from build123d import *

# Parameters (mm, degrees)
F3_D     = 4.5
F3_DEPTH = 7.4
F3_TIP   = 1.3519363928


with BuildPart() as f1:
    # F0 (on Front) → F1 (revolve)
    with BuildSketch(Plane.XZ):
        Polygon((0, 7.5), (-10, 7.5), (-10, 0), (12, 0), (12, 2.5), (0, 2.5), align=None)
    revolve(axis=Axis((1, 0, 0), (1, 0, 0)))

    # F3
    with Locations(Plane(origin=(-10, 0, 0), x_dir=(0, -1, 0), z_dir=(-1, 0, 0))):
        with Locations((0, 0)):
            Hole(F3_D / 2, depth=F3_DEPTH)
            with Locations((0, 0, -(F3_DEPTH + F3_TIP / 2))):  # 118° drill point
                Cone(0, F3_D / 2, F3_TIP, mode=Mode.SUBTRACT)


solid = f1.part
Verification items for the finished model (mm, model axes). A direction names the side the tool comes from. Give positions to 0.01 mm unless a question says otherwise; leave off trailing zeros. Order: outer loops, then holes, each group sorted by start corner. A loop starts at its lowest first (then second) coordinate and runs counter-clockwise, first axis right, second up. Notation, with made-up numbers: M 0.5,65.25 L 17.5,65.25 A14 ccw 17.5,89.25 Z; hole C 7,-4 d10. An arc over 180 degrees is marked long. Use one line per item in the form item = value. Start each with the question number.
Q1. Access from +Z, -Z, +X, -X, +Y, -Y to the whole of each face (thin tool, end or side, straight path). Record for faces 1 (the cylindrical face through (5.92, 2.44, -0.54)), 2 (the cylindrical face through (-6.25, -0.29, 2.23)), 3 (the flat face through (12, 0, 0)).
Q2. Scan lines: line 1 along Z through (x, y) = (-7, 0); line 2 along X through (y, z) = (-3, 4.75). Record each from-to range of solid material in increasing order. Write a range as [from, to].
Q3. Mould release check, pull along Z, two halves, no side actions. Record for faces 4 (the cylindrical face through (-5.07, -0.33, -7.493)), 5 (the conical face through (-1.48, 0.08, -0.38)), 6 (the flat face through (0, -2, 2)): +Z half, -Z half, draft (parallel to the pull), parting line (faces both ways), or undercut.
Q4. Section check A-A (x = -3.75). Enter the section's corners in (y, z), then the cut area to 3 significant figures.
Q5. Go/stop test with flat-tipped pins: pin 1 Ø3.5 at (y, z) = (0, 0) entering from -X; pin 2 Ø1.5 at (y, z) = (5, 3.5) entering from +X; pin 3 Ø5 at (x, y) = (0, -0.5) entering from +Z; pin 4 Ø1 at (x, y) = (9, 2) entering from -Z. Record where each tip stops, or that it passes through.
Q6. Section check C-C (x = 5). Enter the section's corners in (y, z).
Q7. Section check B-B (y = -4.5). Enter the section's corners in (x, z).
Q8. Section check D-D (z = -6.25). Enter the section's corners in (x, y).
Evaluation:
q1.face_1 = +X
q1.face_2 = -X
q1.face_3 = +Z, -Z, +X, +Y, -Y
q2.line_1 = [-7.5, -2.25], [2.25, 7.5]
q2.line_2 = [-10, 0]
q3.face_4 = parting line
q3.face_5 = undercut
q3.face_6 = draft
q4.outline = C 0,0 d15; hole C 0,0 d4.5
q4.area = 161 mm2
q5.pin_1 = -2.3
q5.pin_2 = 0
q5.pin_3 = 7.5
q5.pin_4 = -2
q6.outline = C 0,0 d5
q7.outline = M -10,-6 L 0,-6 L 0,6 L -10,6 Z
q8.outline = M -10,-4.15 L 0,-4.15 L 0,4.15 L -10,4.15 Z
